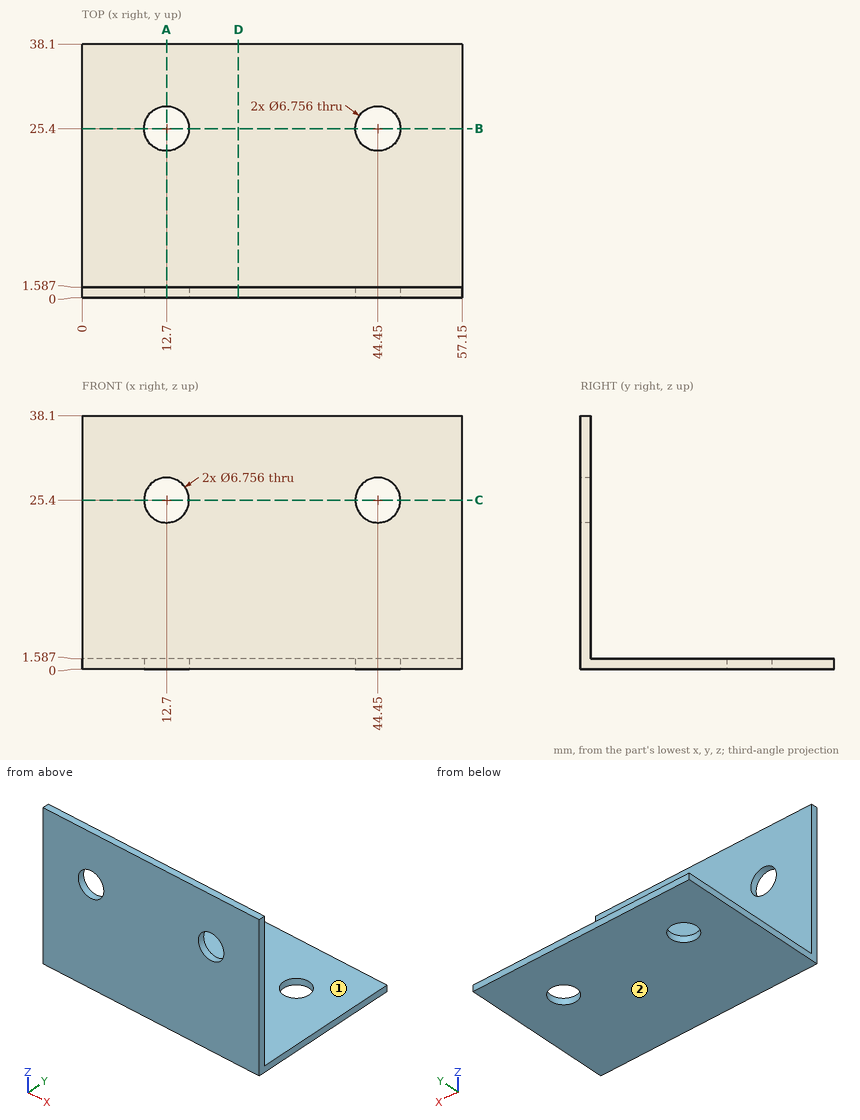
Drawing for the job (mm, zero at the part's lowest x, y, z). A direction names the side the tool comes from. Round coordinates to 2 decimals unless told otherwise and drop trailing zeros. Order: outer loops, then holes, each group sorted by start corner. A loop starts at its lowest first (then second) coordinate and runs counter-clockwise, first axis right, second up. Notation, with made-up numbers: M 46.25,-27.75 L 75.25,-27.75 A30 ccw 75.25,7.25 Z; hole C 45.25,89.25 d6. An arc over 180 degrees is marked long. Use one line per item in the form item = value.
Q1. Saw through at A-A on x = 12.7. Give the cut face in (y, z).
Recorded:
outline = M 0,0 L 22.02,0 L 22.02,1.59 L 1.59,1.59 L 1.59,22.02 L 0,22.02 Z; M 0,28.78 L 1.59,28.78 L 1.59,38.1 L 0,38.1 Z; M 28.78,0 L 38.1,0 L 38.1,1.59 L 28.78,1.59 Z
Q2. Saw through at B-B on y = 25.4. Give the cut face in (x, z).
Recorded:
outline = M 0,0 L 9.32,0 L 9.32,1.59 L 0,1.59 Z; M 16.08,0 L 41.07,0 L 41.07,1.59 L 16.08,1.59 Z; M 47.83,0 L 57.15,0 L 57.15,1.59 L 47.83,1.59 Z
Q3. Probe L1, parallel to X at y = 0.3, z = 25.4; L2, parallel to Z at x = 44.45, y = 1. List the from-to ranges inside material, lowest first.
Recorded:
L1 = 0 to 9.32, 16.08 to 41.07, 47.83 to 57.15
L2 = 0 to 22.02, 28.78 to 38.1
Q4. Flat gauge pins, fed straight in: P1, Ø9, axis at x = 44.45, z = 25.4, coming from the +Y side; P2, Ø5, axis at x = 47.5, y = 29, coming from the +Z side. Where does each tip first touch, or does it go through?
Recorded:
P1 = 1.59
P2 = 1.59
Q5. Which spindle directions (+Z, -Z, +X, -X, +Y, -Y) get a long thin tool onto all of the face, cutting with end or side? Do the marked faces 1 and 2. Say none if no direction does.
Recorded:
face_1 = +Z, +X, -X, +Y
face_2 = -Z, +X, -X, +Y, -Y
Q6. Saw through at D-D on x = 23.5. Give the cut face in (y, z).
Recorded:
outline = M 0,0 L 38.1,0 L 38.1,1.59 L 1.59,1.59 L 1.59,38.1 L 0,38.1 Z
